CAD build for the part. Positions are in the model's coordinates, mm. A direction names the side the tool comes from. Round coordinates to 2 decimals unless told otherwise and drop trailing zeros. Write each loop counter-clockwise with the first axis right and the second up, starting at its lowest first coordinate (ties: lowest second). Pieces come first, ordered by that corner, then holes. Notation, with made-up numbers: (18, 11.25) - (41, 11.25) arc R11 ccw to (41, 22.25) - close; hole circle Ø7 at (-20, 38). An arc over 180 degrees is marked (long way). Use one line per item in the form item = value. Start each with the question number.
Item 1: Band-saw the part on C-C, the plane z = 41.5. List the corners of the cut face in (x, y).
Item 2: Band-saw the part on A-A, the plane y = -68.9. List the corners of the cut face in (x, z), and give its area (3 significant figures).
Item 3: Band-saw the part on D-D, the plane x = 24.5. List the corners of the cut face in (y, z).
Item 4: Tool access for faces 4 (the flat face through (-45.489, -44.75, -18.982)), 5 (the cylindrical face through (69.93, -34.681, 20.975)), 6 (the cylindrical face through (62.59, -42.54, 7.86)): list every direction of +Z, -Z, +X, -X, +Y, -Y with a clear straight run to the whole face (end or side of a thin tool).
Item 5: Band-saw the part on B-B, the plane y = -45.5. List the corners of the cut face in (x, z), and give its area (3 significant figures).
Item 6: Pin check, flat tips, straight feed: pin 1 (1 mm diameter, centred on y = -16, z = -1, fed in from +X); pin 2 (2 mm diameter, centred on y = -5, z = 1.5, fed in from -X); pin 3 (15.5 mm diameter, centred on x = 0, z = 42, fed in from +Y); pin 4 (4 mm diameter, centred on y = -63.9, z = -16.42, fed in from +X). Stop position of each tip, or through.
Item 7: Pull direction Y, two halves, no side cores. Call faces 1 (the flat face through (-38, -71.9, -3)), 2 (the flat face through (65, -50, -29)), 3 (the cylindrical face through (70.07, -56.79, -32.36)): +Y half, -Y half, draft (parallel to the pull), parting line (faces both ways), or undercut.
Item 8: Drill centre lines: L1, parallel to Z at x = 73, y = -58; L2, parallel to X at y = -18.5, z = 32; L3, parallel to X at y = -36.5, z = -9.5. Where is each one in solid material? Low to high.
from build123d import *

# Parameters (mm, degrees)
BOSS_EXTRU_1_DEPTH             = 70
BOSS_EXTRU_2_START             = -45
BOSS_EXTRU_2_DEPTH             = 45
ENL_V_MAT_EXTRU_1_DEPTH        = 15
BOSS_EXTRU_6_START             = -20
BOSS_EXTRU_6_DEPTH             = 20
ESQUISSE10_W                   = 8.2
ESQUISSE10_H                   = 25
ESQUISSE10_R                   = 2.5
BOSS_EXTRU_7_DEPTH             = 10
BOSS_EXTRU_8_DEPTH             = 8
BOSS_EXTRU_8_DIRECTION_2_REACH = 120.835
ESQUISSE12_R                   = 10
ENL_V_MAT_EXTRU_2_DEPTH        = 42.773769853
ESQUISSE13_R                   = 2.25
ENL_V_MAT_EXTRU_3_DEPTH        = 65
CONG_5_R                       = 5
CONG_6_R                       = 50
CONG_7_R                       = 5
CONG_8_R                       = 8
CONG_9_R                       = 8
CONG_10_R                      = 2
CONG_11_R                      = 10


with BuildPart() as part:
    # Esquisse1 → Boss.-Extru.1 (new body)
    with BuildSketch(Plane(origin=(0, 11.1, 0), x_dir=(0, 0, 1), z_dir=(0, -1, 0))):
        with BuildLine():
            Line((-14.419058892, 37.773769853), (-14.419058892, 34.76924835))
            ThreePointArc((-14.419058892, 34.76924835), (18.580941108, -0.173562069), (-14.419058892, -35.116372489))
            Line((-14.419058892, -35.116372489), (-14.419058892, -38.120893991))
            ThreePointArc((-14.419058892, -38.120893991), (21.580941108, -0.173562069), (-14.419058892, 37.773769853))
        make_face()
    extrude(amount=BOSS_EXTRU_1_DEPTH)

    # Esquisse2 → Boss.-Extru.2 (add)
    with BuildSketch(Plane.XZ.offset(58.9).offset(BOSS_EXTRU_2_START)):
        with BuildLine():
            Line((-7.36953704, 20.824754767), (-7.407428488, 53.572216152))
            Line((-7.407428488, 53.572216152), (7.592561471, 53.589572347))
            Line((7.592561471, 53.589572347), (7.630452918, 20.842110962))
            ThreePointArc((7.630452918, 20.842110962), (0.129593041, 21.580915671), (-7.36953704, 20.824754767))
        make_face()
    extrude(amount=BOSS_EXTRU_2_DEPTH)

    # Esquisse3 → Enlèv. mat.-Extru.1 (cut)
    with BuildSketch(Plane(origin=(-7.345431289, 0, -0.008499255), x_dir=(-0.0011570796870464528, 0, 0.999999330583075), z_dir=(-0.999999330583075, 0, -0.0011570796870464528))):
        with BuildLine():
            Line((46.080751274, -28.9), (32.080751274, -28.9))
            ThreePointArc((32.080751274, -28.9), (29.580751274, -26.4), (32.080751274, -23.9))
            Line((32.080751274, -23.9), (46.080751274, -23.9))
            ThreePointArc((46.080751274, -23.9), (48.580751274, -26.4), (46.080751274, -28.9))
        make_face()
        with BuildLine():
            Line((32.080751274, -43.9), (46.080751274, -43.9))
            ThreePointArc((46.080751274, -43.9), (48.580751274, -46.4), (46.080751274, -48.9))
            Line((46.080751274, -48.9), (32.080751274, -48.9))
            ThreePointArc((32.080751274, -48.9), (29.580751274, -46.4), (32.080751274, -43.9))
        make_face()
    extrude(amount=-ENL_V_MAT_EXTRU_1_DEPTH, mode=Mode.SUBTRACT)

    # Esquisse5 → Boss.-Extru.6 (add)
    with BuildSketch(Plane.XZ.offset(52.4).offset(BOSS_EXTRU_6_START)):
        with BuildLine():
            Line((38.120893991, -14.419058892), (65, -14.419058892))
            Line((65, -14.419058892), (65, -35.419058892))
            Line((65, -35.419058892), (75, -35.419058892))
            Line((75, -35.419058892), (75, 23.380941108))
            Line((75, 23.380941108), (65, 23.380941108))
            Line((65, 23.380941108), (65, 5.580941108))
            Line((65, 5.580941108), (31.157428839, 5.580941108))
            ThreePointArc((31.157428839, 5.580941108), (36.060572787, -3.924161464), (38.120893991, -14.419058892))
        make_face()
    extrude(amount=BOSS_EXTRU_6_DEPTH)

    # Esquisse10 → Boss.-Extru.7 (add)
    # profile 1 of 2: a face of its own
    with BuildSketch(Plane(origin=(75, 0, 0), x_dir=(0, 0, -1), z_dir=(1, 0, 0))):
        with Locations((-19.280941108, -64.9)):
            Rectangle(ESQUISSE10_W, ESQUISSE10_H)
        with Locations((-18.980941108, -58.9)):
            Circle(ESQUISSE10_R, mode=Mode.SUBTRACT)
        with Locations((-18.980941108, -68.9)):
            Circle(ESQUISSE10_R, mode=Mode.SUBTRACT)
    # profile 2 of 2: a face of its own
    with BuildSketch(Plane(origin=(75, 0, 0), x_dir=(0, 0, -1), z_dir=(1, 0, 0))):
        with Locations((31.319058892, -64.9)):
            Rectangle(ESQUISSE10_W, ESQUISSE10_H)
        with Locations((31.019058892, -58.9)):
            Circle(ESQUISSE10_R, mode=Mode.SUBTRACT)
        with Locations((31.019058892, -68.9)):
            Circle(ESQUISSE10_R, mode=Mode.SUBTRACT)
    extrude(amount=-BOSS_EXTRU_7_DEPTH)

    # Esquisse11 → Boss.-Extru.8 (add)
    with BuildSketch(Plane(origin=(0, -63.9, 0), x_dir=(0, 0, 1), z_dir=(0, -1, 0))):
        with BuildLine():
            Line((-14.419058892, 37.773769853), (-14.419058892, 42.773769853))
            Line((-14.419058892, 42.773769853), (-23.419058892, 42.773769853))
            Line((-23.419058892, 42.773769853), (-23.419058892, 47.773769853))
            ThreePointArc((-23.419058892, 47.773769853), (-8.548386036, 47.638561364), (5.580941108, 42.999886235))
            ThreePointArc((5.580941108, 42.999886235), (7.341400367, 33.183529475), (12.403351613, 24.590699533))
            Line((12.403351613, 24.590699533), (10.127898152, 22.635626249))
            ThreePointArc((10.127898152, 22.635626249), (-0.909758926, 31.202569218), (-14.419058892, 34.76924835))
            Line((-14.419058892, 34.76924835), (-14.419058892, 37.773769853))
        make_face()
    extrude(amount=BOSS_EXTRU_8_DEPTH)

    # Boss.-Extru.8 direction 2: up to this face of the body (flat: up to its plane)
    boss_extru_8_direction_2_end = Plane(part.part.faces().sort_by_distance((60.159129099, -32.4, -5.026373369))[0])
    # Esquisse11 → Boss.-Extru.8 direction 2 (add, up to the picked face)
    with BuildSketch(Plane(origin=(0, -63.9, 0), x_dir=(0, 0, 1), z_dir=(0, -1, 0)), mode=Mode.PRIVATE) as boss_extru_8_direction_2_sk1:
        with BuildLine():
            Line((-14.419058892, 37.773769853), (-14.419058892, 42.773769853))
            Line((-14.419058892, 42.773769853), (-23.419058892, 42.773769853))
            Line((-23.419058892, 42.773769853), (-23.419058892, 47.773769853))
            ThreePointArc((-23.419058892, 47.773769853), (-8.548386036, 47.638561364), (5.580941108, 42.999886235))
            ThreePointArc((5.580941108, 42.999886235), (7.341400367, 33.183529475), (12.403351613, 24.590699533))
            Line((12.403351613, 24.590699533), (10.127898152, 22.635626249))
            ThreePointArc((10.127898152, 22.635626249), (-0.909758926, 31.202569218), (-14.419058892, 34.76924835))
            Line((-14.419058892, 34.76924835), (-14.419058892, 37.773769853))
        make_face()
    boss_extru_8_direction_2_tool1 = split(extrude(boss_extru_8_direction_2_sk1.sketch, amount=-BOSS_EXTRU_8_DIRECTION_2_REACH, mode=Mode.PRIVATE), bisect_by=boss_extru_8_direction_2_end, keep=Keep.BOTH, mode=Mode.PRIVATE)
    add(boss_extru_8_direction_2_tool1.solids().sort_by(Axis((-38.873879, -63.9, -4.751333), (0, 1, 0)))[0])

    # Esquisse12 → Enlèv. mat.-Extru.2 (cut)
    with BuildSketch(Plane(origin=(0, 0, 0), x_dir=(0, 0, -1), z_dir=(1, 0, 0))):
        with Locations((16.419058892, -63.9)):
            Circle(ESQUISSE12_R)
    extrude(amount=-ENL_V_MAT_EXTRU_2_DEPTH, mode=Mode.SUBTRACT)

    # Esquisse13 → Enlèv. mat.-Extru.3 (cut)
    with BuildSketch(Plane(origin=(0, 0, 0), x_dir=(0, 0, -1), z_dir=(1, 0, 0))):
        with Locations((16.419058892, -63.9)):
            Circle(ESQUISSE13_R)
        Polygon((14.419058892, -32.4), (23.419058892, -32.4), (23.419058892, -56.758571571), align=None)
    extrude(amount=-ENL_V_MAT_EXTRU_3_DEPTH, mode=Mode.SUBTRACT)

    # Congé5
    cong_5_edges = [part.edges().sort_by_distance(p)[0] for p in [
        (-45.273769853, -71.9, -23.419058892),
    ]]
    fillet(cong_5_edges, radius=CONG_5_R)

    # Congé6
    cong_6_edges = [part.edges().sort_by_distance(p)[0] for p in [
        (31.157428839, -42.4, 5.580941108),
    ]]
    fillet(cong_6_edges, radius=CONG_6_R)

    # Congé7
    cong_7_edges = [part.edges().sort_by_distance(p)[0] for p in [
        (7.630452918, -36.4, 20.842110962),
        (-7.36953704, -36.4, 20.824754767),
    ]]
    fillet(cong_7_edges, radius=CONG_7_R)

    # Congé8
    cong_8_edges = [part.edges().sort_by_distance(p)[0] for p in [
        (65, -42.4, 5.580941108),
        (65, -42.4, -14.419058892),
    ]]
    fillet(cong_8_edges, radius=CONG_8_R)

    # Congé9
    cong_9_edges = [part.edges().sort_by_distance(p)[0] for p in [
        (70, -32.4, 23.380941108),
        (70, -32.4, -35.419058892),
    ]]
    fillet(cong_9_edges, radius=CONG_9_R)

    # Congé10
    cong_10_edges = [part.edges().sort_by_distance(p)[0] for p in [
        (70, -77.4, 23.380941108),
        (70, -77.4, -35.419058892),
    ]]
    fillet(cong_10_edges, radius=CONG_10_R)

    # Congé11
    cong_11_edges = [part.edges().sort_by_distance(p)[0] for p in [
        (0.092566491, -13.9, 53.580894249),
        (0.092566491, -58.9, 53.580894249),
    ]]
    fillet(cong_11_edges, radius=CONG_11_R)


solid = part.part
Determined:
q1.outline = (-7.39, -58.9) - (7.61, -58.9) - (7.61, -48.9) - (-7.39, -48.9) - close; (-7.39, -43.9) - (7.61, -43.9) - (7.61, -28.9) - (-7.39, -28.9) - close; (-7.39, -23.9) - (7.61, -23.9) - (7.61, -13.9) - (-7.39, -13.9) - close
q2.outline = (-47.83, -23) - (-42.77, -23) - (-42.77, -7.76) - (-33.74, -7.76) arc R35 cw to (-22.64, 10.13) - (-24.59, 12.4) arc R28.25 cw to (-43, 5.58) arc R48.46 ccw to start; (65, -35.42) - (75, -35.42) - (75, -33.52) - (65, -33.52) - close; (65, -28.52) - (75, -28.52) - (75, -27.22) - (65, -27.22) - close; (65, 15.18) - (75, 15.18) - (75, 16.48) - (65, 16.48) - close; (65, 21.48) - (75, 21.48) - (75, 23.38) - (65, 23.38) - close
q2.area = 380 mm²
q3.outline = (-58.9, 8.74) - (11.1, 8.74) - (11.1, 12.77) - (-32.4, 12.77) - (-32.4, 13.04) - (-52.4, 13.04) - (-52.4, 12.77) - (-58.9, 12.77) - close
q4.face_4 = -Z, -X, +Y
q4.face_5 = +Z, +X, +Y
q4.face_6 = +Z, +Y, -Y
q5.outline = (-48.2, -19.26) - (-42.77, -19.26) - (-42.77, -14.42) - (-34.77, -14.42) arc R35 cw to (35.12, -14.42) - (57, -14.42) arc R8 cw to (65, -22.42) - (65, -35.42) - (75, -35.42) - (75, 23.38) - (65, 23.38) - (65, 13.58) arc R8 cw to (57, 5.58) - (50.77, 5.58) arc R50 cw to (22.02, 14.67) arc R38 ccw to (11.18, 19.95) arc R5 cw to (7.63, 24.73) - (7.62, 29.76) - (-7.38, 29.74) - (-7.37, 24.72) arc R5 cw to (-10.92, 19.93) arc R38 ccw to (-24.59, 12.4) arc R28.25 cw to (-43, 5.58) arc R48.46 ccw to start; (-7.41, 53.57) - (-7.4, 48.4) - (7.6, 48.42) - (7.59, 53.59) - close
q5.area = 2,040 mm²
q6.pin_1 = 35.12
q6.pin_2 = -33.85
q6.pin_3 = -13.9
q6.pin_4 = through
q7.face_1 = -Y half
q7.face_2 = draft
q7.face_3 = undercut
q8.L1 = -35.42 to -33.35, -28.69 to -27.22, 15.18 to 16.65, 21.31 to 23.38
q8.L2 = -7.38 to 7.62
q8.L3 = -47.79 to -34.14, 34.48 to 75
